Verification items for the finished model (mm, model axes). A direction names the side the tool comes from. Give positions to 0.01 mm unless a question says otherwise; leave off trailing zeros. Order: outer loops, then holes, each group sorted by start corner. A loop starts at its lowest first (then second) coordinate and runs counter-clockwise, first axis right, second up. Notation, with made-up numbers: (-12, 78.25) -> (15, 78.25) arc R31 cw to (15, 106.25) -> close; hole circle Ø11 at (-2, -1.5). An arc over 180 degrees is marked (long way). One line per question, with ' | ' between items. Start each with the question number.
Q1. Section check A-A on z = 460.5. Record the cut outline in (x, y), plus the area to 3 significant figures.
Q2. Section check B-B on x = 26. Record the cut outline in (y, z) (1 decimal), plus the area to 3 significant figures.
Q3. Section check C-C on y = 18.5. Record the cut outline in (x, z), plus the area to 3 significant figures.
Q4. Material ranges on probe 1 along X at (y, z) = (22, 219); probe 2 along Y at (x, z) = (36.5, 239.5), recorded low to high. Write a range as [from, to].
Q5. Access from +Z, -Z, +X, -X, +Y, -Y to the whole of each face (thin tool, end or side, straight path). Record for faces 1 (the flat face through (23, 4.762, 278)), 2 (the flat face through (19, 0, 278)), 3 (the flat face through (5, 4.762, 539)), 4 (the flat face through (0, 19, 277)), 5 (the flat face through (5, 4.762, 23)).
Q6. Go/stop test with flat-tipped pins: pin 1 (4 mm diameter, centred on x = 7.5, z = 281, fed in from +Y); pin 2 (2.5 mm diameter, centred on x = 20.5, y = 1.5, fed in from -Z); pin 3 (8 mm diameter, centred on y = 33, z = 58.5, fed in from +X). Record where each tip stops, or that it passes through.
Autodesk Inventor part; units mm, degrees
ref_plane "Start plane" through (0, 0, 0) normal (0, 0, 1) x (1, 0, 0)
ref_plane "End plane" through (0, 0, 561.975) normal (0, 0, 1) x (1, 0, 0)
ref_plane "Work Plane4" through (923.798, 19.05, 561.975) normal (0.7071, 0, -0.7071) x (0, 1, 0)
ref_plane "Start plane" through (0, 0, 0) normal (0, 0, 1) x (1, 0, 0)
ref_plane "End plane" through (0, 0, 561.975) normal (0, 0, 1) x (1, 0, 0)
sketch "Sketch" plane through (0, 0, 0) normal (0, 0, 1) x (1, 0, 0)
  line L0 (38.1, 0) -> (0, 0)
  line L1 (0, 0) -> (0, 38.1)
  line L2 (0, 38.1) -> (2.4765, 38.1)
  line L3 (4.7625, 35.814) -> (4.7625, 9.5885)
  line L4 (9.5885, 4.7625) -> (35.814, 4.7625)
  line L5 (38.1, 2.4765) -> (38.1, 0)
  line L6 (0, -11.0414) -> (0, 31.5385) construction
  line L7 (-11.0414, 0) -> (31.5385, 0) construction
  arc A0 (4.7625, 9.5885) -> (9.5885, 4.7625) centre (9.5885, 9.5885) ccw
  arc A1 (4.7625, 35.814) -> (2.4765, 38.1) centre (2.4765, 35.814) ccw
  arc A2 (38.1, 2.4765) -> (35.814, 4.7625) centre (35.814, 2.4765) ccw
  line L8 (0, 48.4964) -> (0, -20.9644) construction
  line L9 (-20.9644, 0) -> (48.4964, 0) construction
  point P0 (4.7625, 38.1)
  point P1 (4.7625, 4.7625)
  point P2 (38.1, 4.7625)
  dimension "d0" = 38.1
  dimension "d1" = 38.1
  dimension "d2" = 4.7625
  dimension "d3" = 4.7625
  dimension "d10" = 0
  dimension "d11" = 0
  dimension "d14" = 4.826
  dimension "d15" = 2.286
extrude "Body" add sketch "Sketch" along normal up to surface (561.975 mm away) from surface at 0
sketch "Sketch3" plane through (0, 0, 0) normal (0, 0, 1) x (1, 0, 0)
  line L0 (0, 0) -> (10, 0)
ref_plane "Work Plane3" through (0, 0, 0) normal (0, -1, 0) x (1, 0, 0)
sketch "Sketch4" plane through (0, 0, 0) normal (0, -1, 0) x (1, 0, 0)
  line L0 (-2, 0) -> (12, 0)
  line L1 (-2, 561.975) -> (12, 561.975)
  dimension "d17" = 561.975
ref_plane "Work Plane4" through (923.798, 19.05, 561.975) normal (0.7071, 0, -0.7071) x (0, 1, 0)
ref_plane "Work Plane5" through (-130.302, 19.05, 561.975) normal (-0.7071, 0, -0.7071) x (0, 1, 0)
ref_plane "Work Plane6" through (396.748, 0, 561.975) normal (-1, 0, 0) x (0, 1, 0)
sketch "Sketch5" plane through (396.748, 0, 561.975) normal (-1, 0, 0) x (0, 1, 0)
  line L0 (38.1, 0) -> (0, 0)
  line L1 (0, 0) -> (0, 38.1)
  line L2 (0, 38.1) -> (2.4765, 38.1)
  arc A0 (4.7625, 35.814) -> (2.4765, 38.1) centre (2.4765, 35.814) ccw
  line L3 (4.7625, 35.814) -> (4.7625, 9.5885)
  arc A1 (4.7625, 9.5885) -> (9.5885, 4.7625) centre (9.5885, 9.5885) ccw
  line L4 (9.5885, 4.7625) -> (35.814, 4.7625)
  arc A2 (38.1, 2.4765) -> (35.814, 4.7625) centre (35.814, 2.4765) ccw
  line L5 (38.1, 2.4765) -> (38.1, 0)
extrude "Extrusion2" cut sketch "Sketch5" along normal up to surface from surface at -527.05 surface through (-130.302, 19.05, 561.975) normal (-0.7071, 0, -0.7071)
ref_plane "Work Plane7" through (923.798, 19.05, 0) normal (0.7071, 0, 0.7071) x (0.7071, 0, -0.7071)
ref_plane "Work Plane8" through (-130.302, 19.05, 0) normal (-0.7071, 0, 0.7071) x (0.7071, 0, 0.7071)
ref_plane "Work Plane9" through (396.748, 0, 0) normal (-1, 0, 0) x (0, 0, 1)
sketch "Sketch6" plane through (396.748, 0, 0) normal (-1, 0, 0) x (0, 0, 1)
  line L0 (38.1, 0) -> (0, 0)
  line L1 (0, 0) -> (0, 38.1)
  line L2 (0, 38.1) -> (2.4765, 38.1)
  arc A0 (4.7625, 35.814) -> (2.4765, 38.1) centre (2.4765, 35.814) ccw
  line L3 (4.7625, 35.814) -> (4.7625, 9.5885)
  arc A1 (4.7625, 9.5885) -> (9.5885, 4.7625) centre (9.5885, 9.5885) ccw
  line L4 (9.5885, 4.7625) -> (35.814, 4.7625)
  arc A2 (38.1, 2.4765) -> (35.814, 4.7625) centre (35.814, 2.4765) ccw
  line L5 (38.1, 2.4765) -> (38.1, 0)
extrude "Extrusion3" cut sketch "Sketch6" along normal up to surface from surface at -527.05 surface through (-130.302, 19.05, 0) normal (-0.7071, 0, 0.7071)
equation "\"d0\" = G_H"
equation "\"d1\" = G_H"
equation "\"d2\" = G_T"
equation "\"d3\" = G_T"
equation "\"d14\" = G_IR"
equation "\"d15\" = G_ER"
equation "\"d4\" = G_L"
equation "\"G_H\" = 38.1"
equation "\"G_T\" = 4.7625"
equation "\"G_ER\" = 2.286"
equation "\"G_IR\" = 4.826"
equation "\"G_L\" = d17"
equation "\"ex\" = 0"
equation "\"G_OFFSET_START\" = 0"
equation "\"G_OFFSET_END\" = 0"
equation "\"d13\" = G_OFFSET_END + B_L"
equation "\"B_L\" = 561.975"
properties part number "AISC - L 1.5 x 1.5 x 3/16 - 22.125" material "Aluminum 6061-AHC"
Filled in:
1) outline: (0, 0) -> (38.1, 0) -> (38.1, 2.48) arc R2.29 ccw to (35.81, 4.76) -> (9.59, 4.76) arc R4.83 cw to (4.76, 9.59) -> (4.76, 35.81) arc R2.29 ccw to (2.48, 38.1) -> (0, 38.1) -> close | area: 343 mm²
2) outline: (0, 38.1) -> (2.5, 38.1) arc R2.3 cw to (4.8, 35.8) -> (4.8, 526.2) arc R2.3 cw to (2.5, 523.9) -> (0, 523.9) -> close | area: 2,320 mm²
3) outline: (0, 4.76) -> (4.76, 4.76) -> (4.76, 557.21) -> (0, 557.21) -> close | area: 2,630 mm²
4) probe 1: [0, 4.76] | probe 2: [0, 4.66]
5) face 1: +Z, -Z, +X, +Y | face 2: +Z, -Z, +X, -X, -Y | face 3: +Z, +X, -X, -Y | face 4: +Z, -Z, -X, +Y, -Y | face 5: -Z, +X, -X, -Y
6) pin 1: y = 7.02 | pin 2: z = 38.08 | pin 3: x = 4.76
